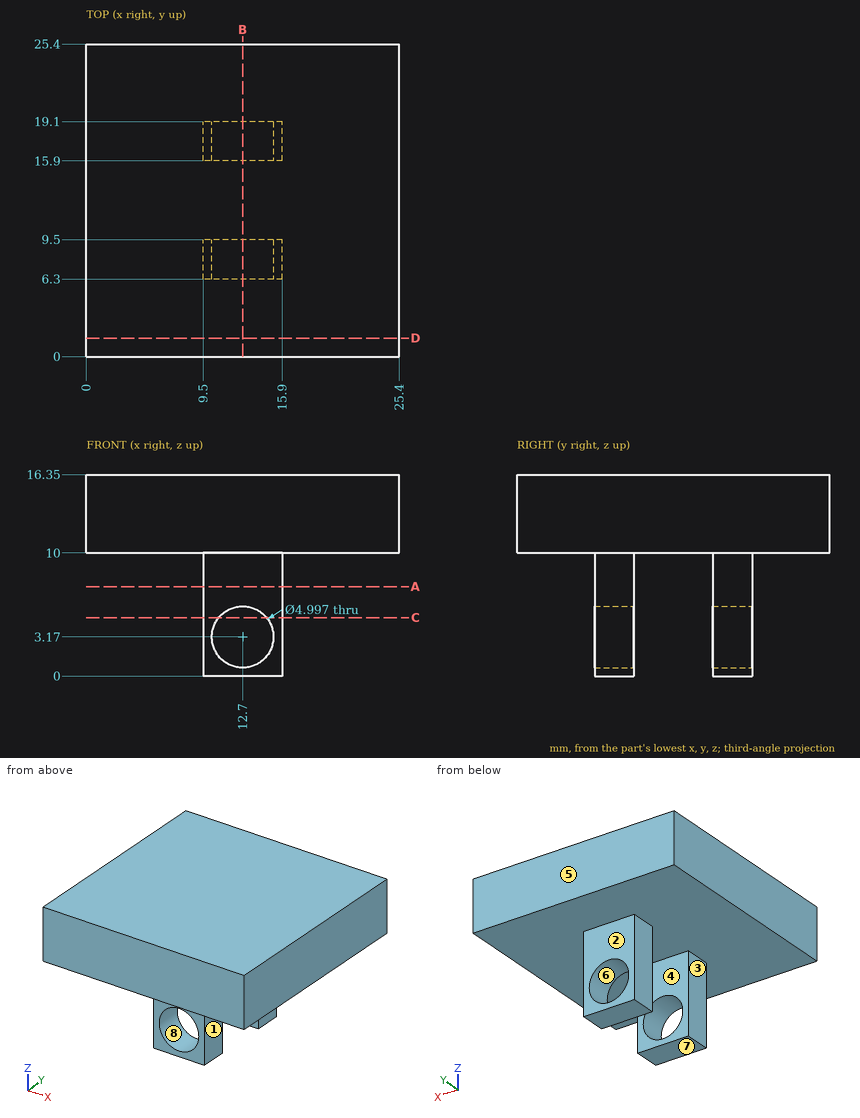
Answer from the drawing. Dimensions are ordinates in mm from the lowest x, y and z of the part. A direction names the side the tool comes from. Give positions to 0.01 mm unless a question says otherwise; leave off trailing zeros. Order: outer loops, then holes, each group sorted by start corner. A loop starts at its lowest first (then second) coordinate and runs counter-clockwise, first axis right, second up. Notation, with made-up numbers: (-26.75, 19) - (-17.75, 19) arc R9 ccw to (-17.75, 36) - close; hole circle Ø8 at (-12, 56). An arc over 180 degrees is marked (long way). Use one line per item in the form item = value.
1) Find section C-C on z = 4.75. Determine the outline of the cut face in (x, y) (1 decimal).
Verdict:
outline = (9.5, 6.3) - (10.8, 6.3) - (10.8, 9.5) - (9.5, 9.5) - close; (9.5, 15.9) - (10.8, 15.9) - (10.8, 19.1) - (9.5, 19.1) - close; (14.6, 6.3) - (15.9, 6.3) - (15.9, 9.5) - (14.6, 9.5) - close; (14.6, 15.9) - (15.9, 15.9) - (15.9, 19.1) - (14.6, 19.1) - close
2) Find section A-A on z = 7.25. Determine the outline of the cut face in (x, y).
Verdict:
outline = (9.5, 6.3) - (15.9, 6.3) - (15.9, 9.5) - (9.5, 9.5) - close; (9.5, 15.9) - (15.9, 15.9) - (15.9, 19.1) - (9.5, 19.1) - close
3) Find section B-B on x = 12.7. Determine the outline of the cut face in (y, z).
Verdict:
outline = (0, 10) - (6.3, 10) - (6.3, 5.67) - (9.5, 5.67) - (9.5, 10) - (15.9, 10) - (15.9, 5.67) - (19.1, 5.67) - (19.1, 10) - (25.4, 10) - (25.4, 16.35) - (0, 16.35) - close; (6.3, 0) - (9.5, 0) - (9.5, 0.67) - (6.3, 0.67) - close; (15.9, 0) - (19.1, 0) - (19.1, 0.67) - (15.9, 0.67) - close
4) The mould has two halves that part along Z. Classify the marked faces 5, 6, 7 and 8: released by +Z, released by -Z, zero draft, split by the parting line, or undercut.
Verdict:
face_5 = zero draft
face_6 = undercut
face_7 = released by -Z
face_8 = undercut
5) Find section D-D on y = 1.5. Determine the outline of the cut face in (x, z).
Verdict:
outline = (0, 10) - (25.4, 10) - (25.4, 16.35) - (0, 16.35) - close
6) Each of these flat-tipped pins is pushed along its axis until it touches: pin 1 (2.5 mm diameter, centred on y = 17, z = 6, fed in from -X); pin 2 (6 mm diameter, centred on x = 4.5, z = 8.5, fed in from +Y); pin 3 (6 mm diameter, centred on x = 7.5, z = 6, fed in from +Y); pin 4 (1.9 mm diameter, centred on x = 11.5, z = 4, fed in from +Y). Where does it stop, or does it pass through?
Verdict:
pin_1 = 9.5
pin_2 = 25.4
pin_3 = 19.1
pin_4 = through
7) Consider probe 1 along Z at (x, y) = (12.7, 17.6); probe 2 along Z at (x, y) = (6, 2.25); probe 3 along X at (y, z) = (9, 6.75). Determine where each line is inside the solid, lowest interval first. Write a range as [from, to].
Verdict:
probe_1 = [0, 0.67], [5.67, 16.35]
probe_2 = [10, 16.35]
probe_3 = [9.5, 15.9]
8) For the marked faces 1, 2, 3 and 4, determine the directions among +Z, -Z, +X, -X, +Y, -Y from which every point of the face is accessible in a straight line to the end or side of a thin tool.
Verdict:
face_1 = -Z, +X, +Y, -Y
face_2 = -Z, +X, -X, +Y
face_3 = -Z, -X, +Y, -Y
face_4 = -Z, +X, -X
